Source: CAD feature listing. Evaluate the final solid. Frame: model axes, mm. A direction names the side the tool comes from. Round coordinates to 2 decimals unless told otherwise and drop trailing zeros. Write each loop counter-clockwise with the first axis right and the second up, starting at its lowest first coordinate (ties: lowest second). Pieces come first, ordered by that corner, then holes. Notation, with made-up numbers: M -33,38 L 11,38 A16 cw 11,53 Z; hole C -11,84.5 d7. An arc over 180 degrees is marked long. Answer in a Markdown table with one row per item. Add a question column.
Item 1: Mould query, pull axis Y, two halves, no side actions, for faces 4 (the face through (-1, 0, 1)), 5 (the face through (-7.8, 12.7, 35.3)), 6 (the face through (37.01, 37.67, -11.65)). Classes: released by +Y, released by -Y, zero draft, split by the parting line, or undercut.
Item 2: Contact query for flat-ended pins moving along their axis: pin 1 (1 mm diameter, centred on x = 3, y = 38.5, fed in from -Z); pin 2 (12 mm diameter, centred on x = 31.5, z = -39.5, fed in from -Y); pin 3 (1.5 mm diameter, centred on y = 22.5, z = -29.5, fed in from -X). Output: stop coordinate, or through.
Item 3: Material intervals for probe 1 along Z at (x, y) = (-1.5, 52); probe 2 along Y at (x, z) = (-8.5, -47.5); probe 3 along X at (y, z) = (12.5, -31), sorted ascending.
Item 4: Cut plane B-B on z = 0. Return loops of the section in (x, y), and give its area (3 significant figures).
Item 5: Cut plane A-A on x = 0. Return loops of the section in (y, z), and give its area (3 significant figures).
Item 6: Cut plane C-C on y = 45. Return loops of the section in (x, z).
Item 7: Set-up query: faces 1 (the face through (37.01, 5.07, -11.65)), 2 (the face through (-50.95, 49.04, 39.06)), 3 (the face through (26, 27.3, -26)). Return all of +Z, -Z, +X, -X, +Y, -Y with unobstructed straight access to the full face (end or side cutting, diameter ignored); none if empty.
Item 8: Cut plane D-D on y = 7.5. Return loops of the section in (x, z).
Autodesk Fusion 360 part; units mm, degrees
sketch "Sketch1" plane through (0, 0, 0) normal (0, 0, 1) x (1, 0, 0)
  line L0 (0, 0) -> (38.8, 0)
  line L1 (38.8, 0) -> (38.8, 10)
  line L2 (38.8, 10) -> (36.15, 10)
  line L3 (36.15, 10) -> (36.15, 15.3)
  line L4 (36.15, 15.3) -> (38.8, 15.3)
  line L5 (38.8, 15.3) -> (38.8, 27.3)
  line L6 (38.8, 27.3) -> (36.15, 27.3)
  line L7 (36.15, 27.3) -> (36.15, 32.6)
  line L8 (36.15, 32.6) -> (38.8, 32.6)
  line L9 (38.8, 32.6) -> (38.8, 42.6)
  line L10 (38.8, 42.6) -> (64.2, 42.6)
  line L11 (64.2, 42.6) -> (64.2, 55.3)
  line L12 (64.2, 55.3) -> (0, 55.3)
  line L13 (0, 55.3) -> (0, 0)
  dimension "d1" = 38.8
  dimension "d2" = 10
  dimension "d3" = 2.65
  dimension "d4" = 5.3
  dimension "d5" = 2.65
  dimension "d7" = 12
  dimension "d8" = 2.65
  dimension "d9" = 5.3
  dimension "d10" = 2.65
  dimension "d11" = 10
  dimension "d12" = 25.4
  dimension "d13" = 12.7
revolve "Revolve1" add sketch "Sketch1" angle 360 about axis through (0, 55.3, 0) along (0, -1, 0)
sketch "Sketch2" plane through (0, 55.3, 0) normal (0, 1, 0) x (-1, 0, 0)
  circle A0 centre (0, 0) radius 64.2
Results below:
| question | item | result |
|---|---|---|
| 1 | face 4 | released by -Y |
| 1 | face 5 | undercut |
| 1 | face 6 | zero draft |
| 2 | pin 1 | z = -38.72 |
| 2 | pin 2 | y = 42.6 |
| 2 | pin 3 | x = -26.06 |
| 3 | probe 1 | -64.18 to 64.18 |
| 3 | probe 2 | 42.6 to 55.3 |
| 3 | probe 3 | -18.6 to 18.6 |
| 4 | outline | M -64.2,42.6 L -38.8,42.6 L -38.8,32.6 L -36.15,32.6 L -36.15,27.3 L -38.8,27.3 L -38.8,15.3 L -36.15,15.3 L -36.15,10 L -38.8,10 L -38.8,0 L 38.8,0 L 38.8,10 L 36.15,10 L 36.15,15.3 L 38.8,15.3 L 38.8,27.3 L 36.15,27.3 L 36.15,32.6 L 38.8,32.6 L 38.8,42.6 L 64.2,42.6 L 64.2,55.3 L -64.2,55.3 Z |
| 4 | area | 4,880 mm2 |
| 5 | outline | M 0,-38.8 L 10,-38.8 L 10,-36.15 L 15.3,-36.15 L 15.3,-38.8 L 27.3,-38.8 L 27.3,-36.15 L 32.6,-36.15 L 32.6,-38.8 L 42.6,-38.8 L 42.6,-64.2 L 55.3,-64.2 L 55.3,64.2 L 42.6,64.2 L 42.6,38.8 L 32.6,38.8 L 32.6,36.15 L 27.3,36.15 L 27.3,38.8 L 15.3,38.8 L 15.3,36.15 L 10,36.15 L 10,38.8 L 0,38.8 Z |
| 5 | area | 4,880 mm2 |
| 6 | outline | C 0,0 d128.4 |
| 7 | face 1 | -Y |
| 7 | face 2 | +Y, -Y |
| 7 | face 3 | none |
| 8 | outline | C 0,0 d77.6 |
